Work out the finished part from the listing and answer in its coordinate system (mm). Face numbers are marked on the shaded views. Give positions to 0.01 mm unless a question says otherwise; leave off trailing zeros. Loops run counter-clockwise (first coordinate to the right, second up) from the corner with the lowest first, then second, coordinate; pieces in that order, holes last.
from build123d import *

# Parameters (mm, degrees)
F0_R         = 2.38125
F1_DEPTH     = 6.35
F2_R         = 4.7625
F3_DEPTH     = 3.175
F4_T1_DEPTH  = 133.35
F4_T3_DEPTH  = 222.25
F4_T6_ANGLE  = 90
F4_T8_ANGLE  = 90
F4_T10_ANGLE = 90
F4_T12_ANGLE = 90
F6_DEPTH     = 0.79375
F8_R         = 4.7625
F9_DEPTH     = 3.175


# Not quite as in the source:
# - a fillet or chamfer that OpenCascade refuses, or shapes differently, is made with other operations: its cross-section is extruded or revolved along the edge and cut away or added


with BuildPart() as f1:
    # F0 (on Front) → F1 (new body)
    with BuildSketch(Plane.XZ):
        with BuildLine():
            Line((123.8407226482, 73.3042017429), (-98.4092773518, 73.3042017429))
            ThreePointArc((-98.4092773518, 73.3042017429), (-102.8994054124, 71.4443298034), (-104.7592773518, 66.9542017429))
            Line((-104.7592773518, 66.9542017429), (-104.7592773518, -66.3957982571))
            ThreePointArc((-104.7592773518, -66.3957982571), (-102.8994054124, -70.8859263176), (-98.4092773518, -72.7457982571))
            Line((-98.4092773518, -72.7457982571), (123.8407226482, -72.7457982571))
            ThreePointArc((123.8407226482, -72.7457982571), (128.3308507087, -70.8859263176), (130.1907226482, -66.3957982571))
            Line((130.1907226482, -66.3957982571), (130.1907226482, 66.9542017429))
            ThreePointArc((130.1907226482, 66.9542017429), (128.3308507087, 71.4443298034), (123.8407226482, 73.3042017429))
        make_face()
        with Locations((-95.8918413821, -60.7033622874)):
            Circle(F0_R, mode=Mode.SUBTRACT)
        with Locations((12.7157226482, -61.6332982571)):
            Circle(F0_R, mode=Mode.SUBTRACT)
        with Locations((-98.4092773518, 0.2792017429)):
            Circle(F0_R, mode=Mode.SUBTRACT)
        with Locations((121.3232866785, -60.7033622874)):
            Circle(F0_R, mode=Mode.SUBTRACT)
        with Locations((123.8407226482, 0.2792017429)):
            Circle(F0_R, mode=Mode.SUBTRACT)
        with Locations((-72.7617797518, 61.2646017429)):
            Circle(F0_R, mode=Mode.SUBTRACT)
        with Locations((12.7157226482, 61.2646017429)):
            Circle(F0_R, mode=Mode.SUBTRACT)
        with Locations((98.1932250482, 61.2646017429)):
            Circle(F0_R, mode=Mode.SUBTRACT)
    extrude(amount=F1_DEPTH)

    # F2 (on face) → F3 (cut)
    with BuildSketch(Plane.XZ.offset(6.35)):
        with Locations((12.7157226482, 61.2646017429)):
            Circle(F2_R)
        with Locations((123.8407226482, 0.2792017429)):
            Circle(F2_R)
        with Locations((121.3232866785, -60.7033622874)):
            Circle(F2_R)
        with Locations((12.7157226482, -61.6332982571)):
            Circle(F2_R)
        with Locations((-95.8918413821, -60.7033622874)):
            Circle(F2_R)
        with Locations((-98.4092773518, 0.2792017429)):
            Circle(F2_R)
    extrude(amount=-F3_DEPTH, mode=Mode.SUBTRACT)

    # F4: fillet of radius 5.08 on 8 edges, made by hand

    # F4_s2 → F4_t1 (cut)
    with BuildSketch(Plane.XY.offset(-66.3957982571)):
        with BuildLine():
            ThreePointArc((-99.6792773518, -6.35), (-103.2713798002, -4.8621024484), (-104.7592773518, -1.27))
            Line((-104.7592773518, -1.27), (-104.7592773518, -6.35))
            Line((-104.7592773518, -6.35), (-99.6792773518, -6.35))
        make_face()
        with BuildLine():
            ThreePointArc((130.1907226482, -1.27), (128.7028250966, -4.8621024484), (125.1107226482, -6.35))
            Line((125.1107226482, -6.35), (130.1907226482, -6.35))
            Line((130.1907226482, -6.35), (130.1907226482, -1.27))
        make_face()
    extrude(amount=F4_T1_DEPTH, mode=Mode.SUBTRACT)

    # F4_s4 → F4_t3 (cut)
    with BuildSketch(Plane.YZ.offset(-98.4092773518)):
        with BuildLine():
            ThreePointArc((-1.27, 73.3042017429), (-4.8621024484, 71.8163041913), (-6.35, 68.2242017429))
            Line((-6.35, 68.2242017429), (-6.35, 73.3042017429))
            Line((-6.35, 73.3042017429), (-1.27, 73.3042017429))
        make_face()
        with BuildLine():
            ThreePointArc((-6.35, -67.6657982571), (-4.8621024484, -71.2579007055), (-1.27, -72.7457982571))
            Line((-1.27, -72.7457982571), (-6.35, -72.7457982571))
            Line((-6.35, -72.7457982571), (-6.35, -67.6657982571))
        make_face()
    extrude(amount=F4_T3_DEPTH, mode=Mode.SUBTRACT)

    # F4_s5 → F4_t6 (revolve, cut)
    with BuildSketch(Plane.YZ.offset(-98.4092773518)):
        with BuildLine():
            ThreePointArc((-6.35, 68.2242017429), (-4.8621024484, 71.8163041913), (-1.27, 73.3042017429))
            Line((-1.27, 73.3042017429), (-6.35, 73.3042017429))
            Line((-6.35, 73.3042017429), (-6.35, 68.2242017429))
        make_face()
    revolve(axis=Axis((-98.4092773518, -6.35, 66.9542017429), (0, -1, 0)), revolution_arc=F4_T6_ANGLE, mode=Mode.SUBTRACT)

    # F4_s7 → F4_t8 (revolve, cut)
    with BuildSketch(Plane.XY.offset(66.9542017429)):
        with BuildLine():
            ThreePointArc((130.1907226482, -1.27), (128.7028250966, -4.8621024484), (125.1107226482, -6.35))
            Line((125.1107226482, -6.35), (130.1907226482, -6.35))
            Line((130.1907226482, -6.35), (130.1907226482, -1.27))
        make_face()
    revolve(axis=Axis((123.8407226482, -6.35, 66.9542017429), (0, -1, 0)), revolution_arc=F4_T8_ANGLE, mode=Mode.SUBTRACT)

    # F4_s9 → F4_t10 (revolve, cut)
    with BuildSketch(Plane.YZ.offset(123.8407226482)):
        with BuildLine():
            ThreePointArc((-6.35, -67.6657982571), (-4.8621024484, -71.2579007055), (-1.27, -72.7457982571))
            Line((-1.27, -72.7457982571), (-6.35, -72.7457982571))
            Line((-6.35, -72.7457982571), (-6.35, -67.6657982571))
        make_face()
    revolve(axis=Axis((123.8407226482, -6.35, -66.3957982571), (0, -1, 0)), revolution_arc=F4_T10_ANGLE, mode=Mode.SUBTRACT)

    # F4_s11 → F4_t12 (revolve, cut)
    with BuildSketch(Plane.XY.offset(-66.3957982571)):
        with BuildLine():
            ThreePointArc((-99.6792773518, -6.35), (-103.2713798002, -4.8621024484), (-104.7592773518, -1.27))
            Line((-104.7592773518, -1.27), (-104.7592773518, -6.35))
            Line((-104.7592773518, -6.35), (-99.6792773518, -6.35))
        make_face()
    revolve(axis=Axis((-98.4092773518, -6.35, -66.3957982571), (0, -1, 0)), revolution_arc=F4_T12_ANGLE, mode=Mode.SUBTRACT)

    # F5 (on face) → F6 (join)
    with BuildSketch(Plane.XZ):
        with BuildLine():
            Line((-92.0592773518, 47.9042017429), (-92.0592773518, -47.3457982571))
            ThreePointArc((-92.0592773518, -47.3457982571), (-90.1994054124, -51.8359263176), (-85.7092773518, -53.6957982571))
            Line((-85.7092773518, -53.6957982571), (111.1407226482, -53.6957982571))
            ThreePointArc((111.1407226482, -53.6957982571), (115.6308507087, -51.8359263176), (117.4907226482, -47.3457982571))
            Line((117.4907226482, -47.3457982571), (117.4907226482, 47.9042017429))
            ThreePointArc((117.4907226482, 47.9042017429), (115.6308507087, 52.3943298034), (111.1407226482, 54.2542017429))
            Line((111.1407226482, 54.2542017429), (-85.7092773518, 54.2542017429))
            ThreePointArc((-85.7092773518, 54.2542017429), (-90.1994054124, 52.3943298034), (-92.0592773518, 47.9042017429))
        make_face()
        with BuildLine():
            ThreePointArc((-88.8842773518, 47.9042017429), (-87.9543413821, 50.1492657732), (-85.7092773518, 51.0792017429))
            Line((-85.7092773518, 51.0792017429), (111.1407226482, 51.0792017429))
            ThreePointArc((111.1407226482, 51.0792017429), (113.3857866785, 50.1492657732), (114.3157226482, 47.9042017429))
            Line((114.3157226482, 47.9042017429), (114.3157226482, -47.3457982571))
            ThreePointArc((114.3157226482, -47.3457982571), (113.3857866785, -49.5908622874), (111.1407226482, -50.5207982571))
            Line((111.1407226482, -50.5207982571), (-85.7092773518, -50.5207982571))
            ThreePointArc((-85.7092773518, -50.5207982571), (-87.9543413821, -49.5908622874), (-88.8842773518, -47.3457982571))
            Line((-88.8842773518, -47.3457982571), (-88.8842773518, 47.9042017429))
        make_face(mode=Mode.SUBTRACT)
    extrude(amount=-F6_DEPTH)

    # F8 (on face) → F9 (cut)
    with BuildSketch(Plane.XZ.offset(6.35)):
        with Locations((-72.7617797518, 61.0206037701)):
            Circle(F8_R)
        with Locations((98.1932250482, 61.0206037701)):
            Circle(F8_R)
    extrude(amount=-F9_DEPTH, mode=Mode.SUBTRACT)


solid = f1.part
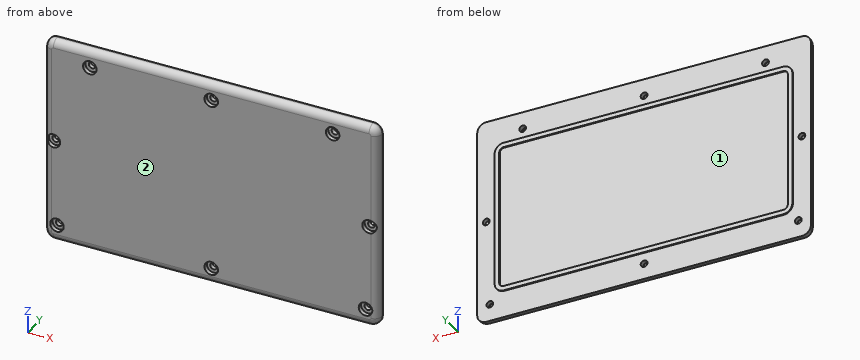
Item 1: Find section A-A, the plane x = 39. Write down the section's boundary in (y, z), plus the area to 3 significant figures.
Item 2: Flat-ended cylindrical pins translate along their axes: pin 1 Ø4 at (y, z) = (-5, -5.5) entering from +X; pin 2 Ø4 at (x, y) = (-47, -5.5) entering from +Z; pin 3 Ø7.5 at (x, z) = (12.72, 61.26) entering from -Y (3 decimals); pin 4 Ø3 at (x, z) = (121.5, -61) entering from -Y. Find the tip coordinate at first contact, or state that the pin passes through.
Item 3: Determine the mould class of the marked faces 1 and 2 for opening direction Z: released by +Z, released by -Z, zero draft, split by the parting line, or undercut.
Item 4: Consider line 1 (X direction, y = -3, z = 63); line 2 (Y direction, x = 1.5, z = -5); line 3 (X direction, y = -5, z = -55). Determine where each line is inside the solid, lowest interval first.
Item 5: Find section B-B, the plane z = -25. Write down the section's boundary in (x, y), plus the area to 3 significant figures.
Ans:
1. outline: (-6.35, -67.67) arc R5.08 ccw to (-1.27, -72.75) - (0, -72.75) - (0, -53.7) - (0.79, -53.7) - (0.79, -50.52) - (0, -50.52) - (0, 51.08) - (0.79, 51.08) - (0.79, 54.25) - (0, 54.25) - (0, 73.3) - (-1.27, 73.3) arc R5.08 ccw to (-6.35, 68.22) - close
1. area: 921 mm2
2. pin 1: stops at x = 129.89
2. pin 2: stops at z = 72.79
2. pin 3: stops at y = -3.175
2. pin 4: passes through
3. face 1: undercut
3. face 2: zero draft
4. line 1: x = -104.46 to -74.39, -71.13 to 11.09, 14.35 to 96.56, 99.82 to 129.89
4. line 2: y = -6.35 to 0
4. line 3: x = -103.13 to 128.56
5. outline: (-104.76, -1.27) arc R5.08 ccw to (-99.68, -6.35) - (125.11, -6.35) arc R5.08 ccw to (130.19, -1.27) - (130.19, 0) - (117.49, 0) - (117.49, 0.79) - (114.32, 0.79) - (114.32, 0) - (-88.88, 0) - (-88.88, 0.79) - (-92.06, 0.79) - (-92.06, 0) - (-104.76, 0) - close
5. area: 1,490 mm2
